Verification items for this drawing (mm, ordinates from the low corner). Round coordinates to 2 decimals unless told otherwise and drop trailing zeros. Loops run counter-clockwise (first coordinate to the right, second up) from the corner with the lowest first, then second, coordinate; pieces in that order, holes last. Notation, with made-up numbers: (72.25, -3.5) -> (84.25, -3.5) arc R21 ccw to (84.25, 21.5) -> close; hole circle Ø10 at (75.25, 66). An arc over 180 degrees is marked (long way). Use a Markdown table: item, result. Add a question column.
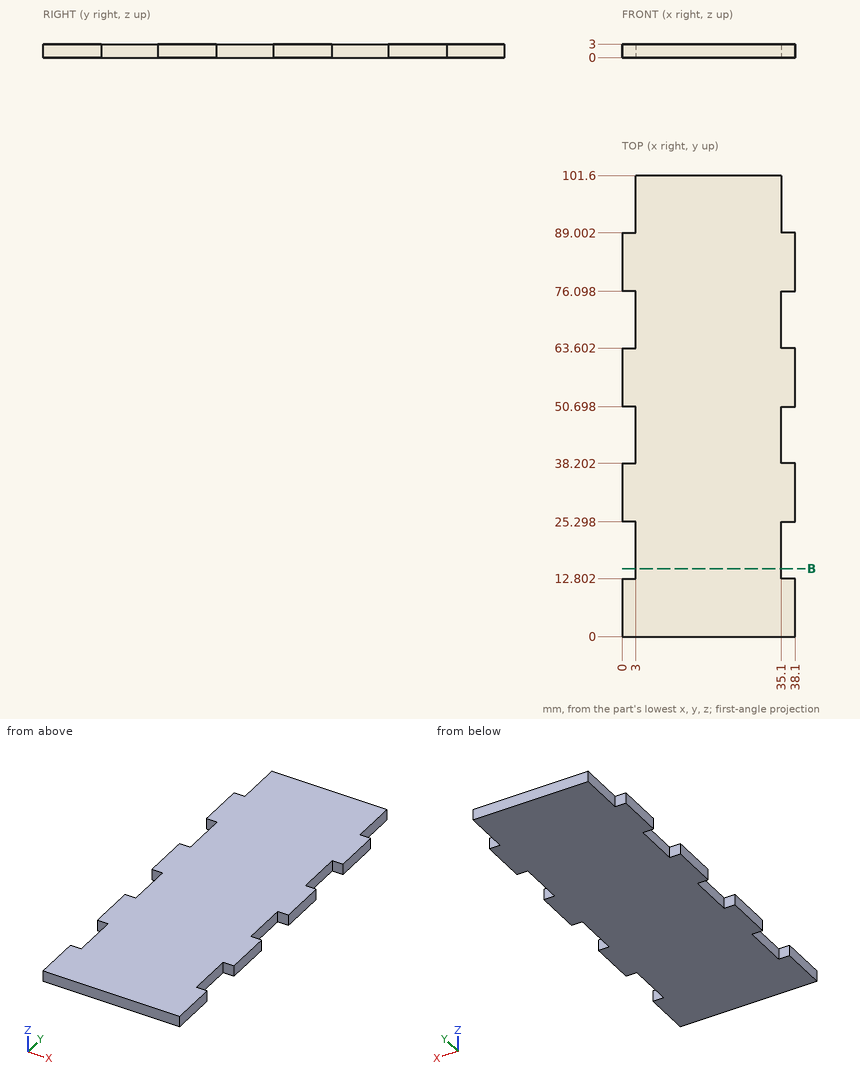
1) Go/stop test with flat-tipped pins: pin 1 (0.9 mm diameter, centred on x = 1, z = 2, fed in from +Y); pin 2 (1.5 mm diameter, centred on y = 20, z = 2, fed in from +X); pin 3 (1.5 mm diameter, centred on y = 97.5, z = 2, fed in from -X). Record where each tip stops, or that it passes through.
2) Sectioned sample at B-B on y = 15. Enter the section's corners in (x, z).
3) Thickness scan on line 1 (X direction, y = 89.5, z = 2.8). Record the ranges inside material, lowest first.
Geometry results:
| question | item | result |
|---|---|---|
| 1 | pin 1 | y = 89 |
| 1 | pin 2 | x = 35.1 |
| 1 | pin 3 | x = 3 |
| 2 | outline | (3, 0) -> (35.1, 0) -> (35.1, 3) -> (3, 3) -> close |
| 3 | line 1 | 3 to 35.1 |
